Check sheet for the modelled part. Datum: model origin and axes. Units: mm. A direction names the side the tool comes from. Give positions to 0.01 mm unless a question says otherwise; leave off trailing zeros. Loops run counter-clockwise (first coordinate to the right, second up) from the corner with the lowest first, then second, coordinate; pieces in that order, holes last. Notation, with made-up numbers: (-27, -33) - (-3, -33) arc R11 ccw to (-3, -27) - close; hole circle Ø3 at (-24.75, -23.5). An arc over 180 degrees is marked (long way). Use one line per item in the form item = value.
from build123d import *

# Parameters (mm, degrees)
BOSS_EXTRUDE1_DEPTH = 6


with BuildPart() as part:
    # Sketch6 → Boss-Extrude1 (new body)
    with BuildSketch(Plane.XY):
        with BuildLine():
            Line((-18.05, -1.259488518), (18.05, -1.259488518))
            ThreePointArc((18.05, -1.259488518), (18.403553391, -1.113041908), (18.55, -0.759488518))
            Line((18.55, -0.759488518), (18.55, 2.990511482))
            ThreePointArc((18.55, 2.990511482), (18.403553391, 3.344064873), (18.05, 3.490511482))
            Line((18.05, 3.490511482), (17.55, 3.490511482))
            ThreePointArc((17.55, 3.490511482), (17.196446609, 3.636958092), (17.05, 3.990511482))
            Line((17.05, 3.990511482), (17.05, 5.960429817))
            ThreePointArc((17.05, 5.960429817), (17.196446609, 6.313983207), (17.55, 6.460429817))
            Line((17.55, 6.460429817), (20.6, 6.460429817))
            ThreePointArc((20.6, 6.460429817), (21.307106781, 6.753323035), (21.6, 7.460429817))
            Line((21.6, 7.460429817), (21.6, 16.490511482))
            Line((21.6, 16.490511482), (-21.6, 16.490511482))
            Line((-21.6, 16.490511482), (-21.6, 7.460429817))
            ThreePointArc((-21.6, 7.460429817), (-21.307106781, 6.753323035), (-20.6, 6.460429817))
            Line((-20.6, 6.460429817), (-17.55, 6.460429817))
            ThreePointArc((-17.55, 6.460429817), (-17.196446609, 6.313983207), (-17.05, 5.960429817))
            Line((-17.05, 5.960429817), (-17.05, 5.25))
            ThreePointArc((-17.05, 5.25), (-17.196446609, 4.896446609), (-17.55, 4.75))
            Line((-17.55, 4.75), (-18.05, 4.75))
            ThreePointArc((-18.05, 4.75), (-18.403553391, 4.603553391), (-18.55, 4.25))
            Line((-18.55, 4.25), (-18.55, -0.759488518))
            ThreePointArc((-18.55, -0.759488518), (-18.403553391, -1.113041908), (-18.05, -1.259488518))
        make_face()
    extrude(amount=BOSS_EXTRUDE1_DEPTH)


solid = part.part
Item 1: Section check B-B on y = 0. Record the boundary of the cut face in (x, z), then the cut area to 3 significant figures.
Answer block:
outline = (-18.55, 0) - (18.55, 0) - (18.55, 6) - (-18.55, 6) - close
area = 223 mm2
Item 2: Thickness scan on L1, parallel to X at y = 2, z = 3.8; L2, parallel to X at y = 3.25, z = 1.55. Record the ranges inside material, lowest first.
Answer block:
L1 = -18.55 to 18.55
L2 = -18.55 to 18.48
Item 3: Access from +Z, -Z, +X, -X, +Y, -Y to the whole of each face (thin tool, end or side, straight path). Record for faces 1 (the face through (-18.55, 2, 3)), 2 (the face through (17.05, 5, 3)), 3 (the face through (18.55, 1, 3)), 4 (the face through (-19, 6.46, 3)).
Answer block:
face_1 = +Z, -Z, -X, -Y
face_2 = +Z, -Z, +X
face_3 = +Z, -Z, +X, -Y
face_4 = +Z, -Z, -X
Item 4: Gauge pin test, flat ends, axial feed: P1, Ø3, axis at y = 0, z = 3, coming from the +X side; P2, Ø0.9, axis at x = -18.5, z = 1.5, coming from the -Y side; P3, Ø0.6, axis at y = 5, z = 3.5, coming from the +X side. Record the tip position at first contact, or that the pin passes through.
Answer block:
P1 = 18.55
P2 = -1.26
P3 = 17.05
Item 5: Section check A-A on z = 2. Record the boundary of the cut face in (x, y), then the cut area to 3 significant figures.
Answer block:
outline = (-21.6, 7.46) arc R1 ccw to (-20.6, 6.46) - (-17.55, 6.46) arc R0.5 cw to (-17.05, 5.96) - (-17.05, 5.25) arc R0.5 cw to (-17.55, 4.75) - (-18.05, 4.75) arc R0.5 ccw to (-18.55, 4.25) - (-18.55, -0.76) arc R0.5 ccw to (-18.05, -1.26) - (18.05, -1.26) arc R0.5 ccw to (18.55, -0.76) - (18.55, 2.99) arc R0.5 ccw to (18.05, 3.49) - (17.55, 3.49) arc R0.5 cw to (17.05, 3.99) - (17.05, 5.96) arc R0.5 cw to (17.55, 6.46) - (20.6, 6.46) arc R1 ccw to (21.6, 7.46) - (21.6, 16.49) - (-21.6, 16.49) - close
area = 712 mm2
Item 6: Mould release check, pull along Y, two halves, no side actions. Record for faces 5 (the face through (0, -1.259, 3)), 6 (the face through (19, 6.46, 3)), 7 (the face through (0, 16.491, 3)), 8 (the face through (-21.6, 12, 3)): released by +Y, released by -Y, zero draft, split by the parting line, or undercut.
Answer block:
face_5 = released by -Y
face_6 = undercut
face_7 = released by +Y
face_8 = zero draft
